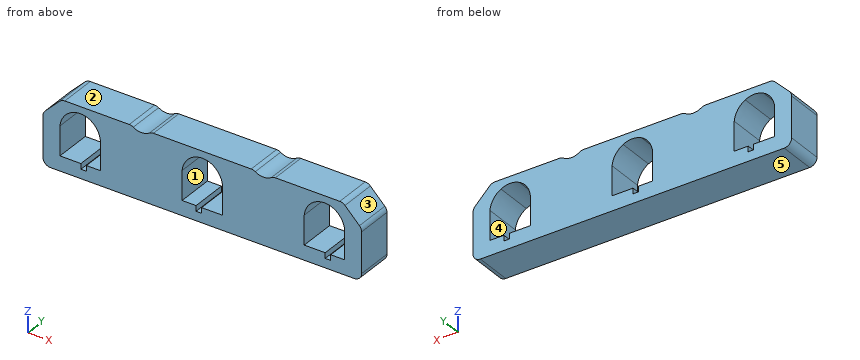
from build123d import *

# Parameters (mm, degrees)
F0_W      = 79.248
F0_H      = 56.769
F1_DEPTH  = 25.4
F2_W      = 2.55016
F2_H      = 56.769
F3_DEPTH  = 25.4
F7_W      = 84.34832
F7_H      = 56.769
F8_DEPTH  = 25.4010001
F10_DEPTH = 25.4010001
F12_DEPTH = 25.4010001
F13_R     = 10.16
F14_R     = 5.08


with BuildPart() as f1:
    # F0 (on Front) → F1 (new body)
    with BuildSketch(Plane.XZ):
        with Locations((-65.9926355079, 23.2293278964)):
            Rectangle(F0_W, F0_H)
        with BuildLine():
            Line((-52.0226355079, 25.0708278964), (-52.0226355079, 5.0048278964))
            Line((-52.0226355079, 5.0048278964), (-66.5006355079, 5.0048278964))
            Line((-66.5006355079, 5.0048278964), (-66.5006355079, 1.1948278964))
            Line((-66.5006355079, 1.1948278964), (-70.3106355079, 1.1948278964))
            Line((-70.3106355079, 1.1948278964), (-70.3106355079, 5.0048278964))
            Line((-70.3106355079, 5.0048278964), (-79.9626355079, 5.0048278964))
            Line((-79.9626355079, 5.0048278964), (-79.9626355079, 25.0708278964))
            add(Edge.make_bspline(
                [(-72.3426355079, 36.6816155863), (-79.143780816, 33.0532444332), (-79.9626355079, 25.0708278964)],
                knots=[0.4689121613, 0.4689121613, 0.4689121613, 1.4631850988, 1.4631850988, 1.4631850988], degree=2, weights=[1, 0.878951812, 1]))
            add(Edge.make_bspline(
                [(-65.9926355079, 38.2788278964), (-69.3487651043, 38.2788278964), (-72.3426355079, 36.6816155863)],
                knots=[0, 0, 0, 0.4689121613, 0.4689121613, 0.4689121613], degree=2, weights=[1, 0.9726408453, 1]))
            add(Edge.make_bspline(
                [(-59.6426355079, 36.6816155863), (-62.6365059115, 38.2788278964), (-65.9926355079, 38.2788278964)],
                knots=[5.8142731459, 5.8142731459, 5.8142731459, 6.2831853072, 6.2831853072, 6.2831853072], degree=2, weights=[1, 0.9726408453, 1]))
            add(Edge.make_bspline(
                [(-52.0226355079, 25.0708278964), (-52.8414901998, 33.0532444332), (-59.6426355079, 36.6816155863)],
                knots=[4.8200002084, 4.8200002084, 4.8200002084, 5.8142731459, 5.8142731459, 5.8142731459], degree=2, weights=[1, 0.878951812, 1]))
        make_face(mode=Mode.SUBTRACT)
    extrude(amount=F1_DEPTH)

    # F2 (on face) → F3 (join, through all)
    with BuildSketch(Plane.XZ.offset(25.4)):
        with Locations((-106.8917155079, 23.2293278964)):
            Rectangle(F2_W, F2_H)
        with Locations((-25.0935555079, 23.2293278964)):
            Rectangle(F2_W, F2_H)
    extrude(amount=-F3_DEPTH)

    # F4: F1 across face


with BuildPart() as f1_1:
    add(f1.part)
    add(f1.part.mirror(Plane(origin=(-108.1667955079, -12.7, 23.2293278964), x_dir=(0, -1, 0), z_dir=(-1, 0, 0))))

    # F5: F1 across face


with BuildPart() as f1_2:
    add(f1_1.part)
    add(f1_1.part.mirror(Plane(origin=(-23.8184755079, -12.7, 23.2293278964), x_dir=(0, 1, 0), z_dir=(1, 0, 0))))

    # F7 (on face) → F8 (cut, through all)
    with BuildSketch(Plane.XZ.offset(25.4)):
        with Locations((102.7040044921, 23.2293278964)):
            Rectangle(F7_W, F7_H)
    extrude(amount=-F8_DEPTH, mode=Mode.SUBTRACT)

    # F9 (on face) → F10 (cut, through all)
    with BuildSketch(Plane.XZ.offset(25.4)):
        Polygon((60.5298444921, -5.1551721036), (60.5298444921, 51.6138278964), (44.0198444921, 51.6138278964), (-176.0051155079, 51.6138278964), (-192.5151155079, 51.6138278964), (-192.5151155079, -5.1551721036), (-176.0051155079, -5.1551721036), (-176.0051155079, 30.0238278964), (-163.0204147545, 43.0085286498), (-133.5769593716, 43.0085286498), (31.0351437387, 43.0085286498), (44.0198444921, 30.0238278964), (44.0198444921, -5.1551721036), align=None)
    extrude(amount=-F10_DEPTH, mode=Mode.SUBTRACT)

    # F11 (on face) → F12 (cut, through all)
    with BuildSketch(Plane.XZ.offset(25.4)):
        Polygon((-30.6416433652, 43.0085286498), (-23.8847362613, 38.2790486498), (-17.1278291575, 43.0085286498), align=None)
        Polygon((-114.8574418583, 43.0085286498), (-108.1005347545, 38.2790486498), (-101.3436276506, 43.0085286498), align=None)
    extrude(amount=-F12_DEPTH, mode=Mode.SUBTRACT)

    # F13
    f13_edges = [f1_2.edges().sort_by_distance(p)[0] for p in [
        (-23.884736, -12.7, 38.279049),
        (-108.100535, -12.7, 38.279049),
    ]]
    fillet(f13_edges, radius=F13_R)

    # F14
    f14_edges = [f1_2.edges().sort_by_distance(p)[0] for p in [
        (-17.127829, -12.7, 43.008529),
        (-30.641643, -12.7, 43.008529),
        (-101.343628, -12.7, 43.008529),
        (-114.857442, -12.7, 43.008529),
        (-163.020415, -12.7, 43.008529),
        (-176.005116, -12.7, 30.023828),
        (31.035144, -12.7, 43.008529),
        (44.019844, -12.7, 30.023828),
        (44.019844, -12.7, -5.155172),
        (-176.005116, -12.7, -5.155172),
    ]]
    fillet(f14_edges, radius=F14_R)


solid = f1_2.part
CAD build for the part. Positions are in the model's coordinates, mm. Face numbers are marked on the shaded views. A direction names the side the tool comes from. Coordinates: 2 decimals unless noted, no trailing zeros. Write each loop counter-clockwise with the first axis right and the second up, starting at its lowest first coordinate (ties: lowest second). Pieces come first, ordered by that corner, then holes. Notation, with made-up numbers: M -38,-18.75 L -13,-18.75 A22 cw -13,20.25 Z; hole C 0,62 d2. An arc over 180 degrees is marked long. Answer as a JSON object with one key per item and string values. Group by question number.
1) Pin check, flat tips, straight feed: pin 1 Ø2 at (x, z) = (-108, 15) entering from +Y; pin 2 Ø1 at (x, y) = (-113.5, -5.5) entering from +Z; pin 3 Ø4 at (x, y) = (-105.5, -12) entering from +Z; pin 4 Ø3 at (y, z) = (-2.5, 36.5) entering from +X. Stop position of each tip, or through.
2) Mould opens along Z. For the marked faces 3, 4 and 5 say: +Z half, -Z half, draft (parallel to the pull), parting line (faces both ways), or undercut.
3) Saw through at C-C (x = -25.5). Write the cut outline in (y, z), plus the area to 3 significant figures.
4) Saw through at B-B (y = -21.5). Give the number of separate pieces and of enclosed holes in the cut face, plus the area to 3 significant figures.
5) Wall check: line 1 (X direction, y = -14, z = 20); line 2 (X direction, y = -10.5, z = 35); line 3 (Z direction, x = 20.5, y = -18). Give the ranges that are in metal, low to high. Write a range as from..to.
6) Saw through at A-A (z = 19). Write the cut outline in (x, y).
7) Tool access for the marked faces 1 and 2: list every direction of +Z, -Z, +X, -X, +Y, -Y with a clear straight run to the whole face (end or side of a thin tool).
Values follow:
{
 "1": {"pin 1": "stops at y = 0", "pin 2": "stops at z = 42.38", "pin 3": "stops at z = 41.62", "pin 4": "stops at x = 39.04"},
 "2": {"face 3": "+Z half", "face 4": "undercut", "face 5": "-Z half"},
 "3": {"outline": "M -25.4,-5.16 L 0,-5.16 L 0,40.65 L -25.4,40.65 Z", "area": "1,160 mm2"},
 "4": {"separate pieces": "1", "enclosed holes": "3", "area": "7,800 mm2"},
 "5": {"line 1": "x = -176.01..-164.31, -136.37..-79.96, -52.02..4.39, 32.33..44.02", "line 2": "x = -171.03..-159.16, -141.52..-74.81, -57.17..9.54, 27.18..39.04", "line 3": "z = -5.16..1.19, 38.11..43.01"},
 "6": {"outline": "M -176.01,-25.4 L -164.31,-25.4 L -164.31,0 L -176.01,0 Z; M -136.37,-25.4 L -79.96,-25.4 L -79.96,0 L -136.37,0 Z; M -52.02,-25.4 L 4.39,-25.4 L 4.39,0 L -52.02,0 Z; M 32.33,-25.4 L 44.02,-25.4 L 44.02,0 L 32.33,0 Z"},
 "7": {"face 1": "+Y, -Y", "face 2": "+Z, +X, -X, +Y, -Y"}
}
